Here's how the part is built. I have some questions about the finished solid (model axes, mm). Coordinates: 2 decimals unless noted, no trailing zeros. Write each loop counter-clockwise with the first axis right and the second up, starting at its lowest first coordinate (ties: lowest second). Pieces come first, ordered by that corner, then holes. Notation, with made-up numbers: M -8.75,-7 L 32.25,-7 A17 cw 32.25,22 Z; hole C 68,31.25 d2. An arc over 180 degrees is marked long. Use one line per item in the form item = value. Start each with the question number.
1. I want a section at A-A, the plane x = 0. List the corners of the cut face in (y, z) for me, plus the area to 3 significant figures.
2. I'm going to push flat-ended pins straight in: pin 1 Ø1.5 at (x, z) = (-3, 2) entering from -Y; pin 2 Ø3 at (y, z) = (-2.5, 1.5) entering from -X. Where does each tip first touch, or does it pass through?
3. I want a section at C-C, the plane z = 7.5. List the corners of the cut face in (x, y) for me, plus the area to 3 significant figures.
4. Please list where these lines run through material, in increasing order: line 1 along X through (y, z) = (-0.5, 6.5); line 2 along Y through (x, z) = (-0.5, 5.5); line 3 along Y through (x, z) = (2.25, 2.75). Write a range as [from, to].
5. I want a section at B-B, the plane y = 0. List the corners of the cut face in (x, z) for me, plus the area to 3 significant figures.
from build123d import *

# Parameters (mm, degrees)
F0_R     = 4
F0_W     = 2.8
F0_H     = 1.4
F1_DEPTH = 9
F2_SIZE  = 0.5


with BuildPart() as f1:
    # F0 (on Top) → F1 (new body)
    with BuildSketch(Plane.XY):
        Circle(F0_R)
        Rectangle(F0_W, F0_H, mode=Mode.SUBTRACT)
    extrude(amount=F1_DEPTH)

    # F2
    f2_edges = [f1.edges().sort_by_distance(p)[0] for p in [
        (-4, 0, 9),
        (-4, 0, 0),
        (1.4, 0, 0),
        (0, 0.7, 0),
        (-1.4, 0, 0),
        (0, -0.7, 0),
        (0, 0.7, 9),
        (1.4, 0, 9),
        (-1.4, 0, 9),
        (0, -0.7, 9),
    ]]
    chamfer(f2_edges, length=F2_SIZE)


solid = f1.part
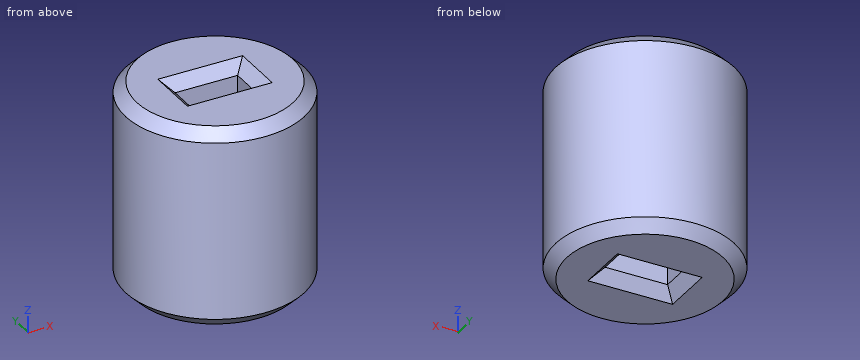
Answer list:
q1.outline = M -4,0.5 L -3.5,0 L -1.2,0 L -0.7,0.5 L -0.7,8.5 L -1.2,9 L -3.5,9 L -4,8.5 Z; M 0.7,0.5 L 1.2,0 L 3.5,0 L 4,0.5 L 4,8.5 L 3.5,9 L 1.2,9 L 0.7,8.5 Z
q1.area = 58.4 mm²
q2.pin_1 = -3.31
q2.pin_2 = -3.87
q3.outline = C 0,0 d8; hole M -1.4,-0.7 L 1.4,-0.7 L 1.4,0.7 L -1.4,0.7 Z
q3.area = 46.3 mm²
q4.line_1 = [-3.97, -1.4], [1.4, 3.97]
q4.line_2 = [-3.97, -0.7], [0.7, 3.97]
q4.line_3 = [-3.31, 3.31]
q5.outline = M -4,0.5 L -3.5,0 L -1.9,0 L -1.4,0.5 L -1.4,8.5 L -1.9,9 L -3.5,9 L -4,8.5 Z; M 1.4,0.5 L 1.9,0 L 3.5,0 L 4,0.5 L 4,8.5 L 3.5,9 L 1.9,9 L 1.4,8.5 Z
q5.area = 45.8 mm²
